The listing builds one solid part. Answer for the finished solid, in the listing's coordinates (mm). Face numbers are marked on the shaded views. A direction names the side the tool comes from. Round coordinates to 2 decimals unless told otherwise and drop trailing zeros. Write each loop counter-clockwise with the first axis right and the second up, starting at its lowest first coordinate (ties: lowest second). Pieces come first, ordered by that corner, then holes. Notation, with made-up numbers: (34, 75.25) - (55, 75.25) arc R6 ccw to (55, 85.25) - close; hole circle Ø8 at (-3, 50). An arc over 180 degrees is marked (long way). Return JSON: item names as keys, results as strings. Group by question number.
(1) Section C-C, the plane x = 14.5 is taken. Write down the section's boundary in (y, z).
(2) Determine the mould class of the marked faces 3, 4, 5 and 6 for opening direction Z: +Z half, -Z half, draft (parallel to the pull), parting line (faces both ways), or undercut.
(3) Find the intervals of material crossed by line 1 along X through (y, z) = (-4.5, -2.5); line 2 along Y through (x, z) = (13, 1.25), in increasing order. Write a range as [from, to].
(4) Section A-A, the plane y = -3 is taken. Give the number of separate pieces and of enclosed holes in the cut face, then the cut area to 3 significant figures.
(5) Section D-D, the plane z = 6 is taken. Write down the section's boundary in (x, y), then the cut area to 3 significant figures.
(6) Section B-B, the plane z = 0 is taken. Write down the section's boundary in (x, y), then the cut area to 3 significant figures.
(7) Which of the six approach directions +Z, -Z, +X, -X, +Y, -Y give full straight-line access (tool end or side, diameter ignored) to the marked faces 1 and 2?
```python
from build123d import *

# Parameters (mm, degrees)
SKETCH2_W           = 42
SKETCH2_H           = 17.8
BOSS_EXTRUDE1_DEPTH = 2
SKETCH3_W           = 2
SKETCH3_H           = 17.8
BOSS_EXTRUDE2_DEPTH = 10
BOSS_EXTRUDE3_DEPTH = 2
SKETCH5_R           = 2.5
CUT_EXTRUDE1_DEPTH  = 2
SKETCH6_R           = 1.25
CUT_EXTRUDE2_DEPTH  = 2


with BuildPart() as part:
    # Sketch2 → Boss-Extrude1 (new body)
    with BuildSketch(Plane(origin=(0, 0, 0), x_dir=(1, 0, 0), z_dir=(0, 1, 0))):
        Rectangle(SKETCH2_W, SKETCH2_H)
    extrude(amount=BOSS_EXTRUDE1_DEPTH)

    # Sketch3 → Boss-Extrude2 (add)
    with BuildSketch(Plane.XZ):
        with Locations((-20, 0)):
            Rectangle(SKETCH3_W, SKETCH3_H)
        with Locations((20, 0)):
            Rectangle(SKETCH3_W, SKETCH3_H)
    extrude(amount=BOSS_EXTRUDE2_DEPTH)

    # Sketch4 → Boss-Extrude3 (add)
    with BuildSketch(Plane.XY.offset(8.9)):
        Polygon((-19, 0), (-14, 0), (-19, -5), align=None)
        Polygon((19, -5), (14, 0), (19, 0), align=None)
    boss_extrude3 = extrude(amount=-BOSS_EXTRUDE3_DEPTH)

    # Mirror1: Boss-Extrude3 across plane
    add(boss_extrude3.mirror(Plane.XY))

    # Sketch5 → Cut-Extrude1 (cut)
    with BuildSketch(Plane.XZ):
        with Locations((-8.319906625, 0)):
            Circle(SKETCH5_R)
        with Locations((6.680093375, 0)):
            Circle(SKETCH5_R)
    extrude(amount=-CUT_EXTRUDE1_DEPTH, mode=Mode.SUBTRACT)

    # Sketch6 → Cut-Extrude2 (cut)
    with BuildSketch(Plane(origin=(-19, 0, 0), x_dir=(0, 0, -1), z_dir=(1, 0, 0))):
        with Locations((-4, -3)):
            Circle(SKETCH6_R)
        with Locations((4, -3)):
            Circle(SKETCH6_R)
    cut_extrude2 = extrude(amount=-CUT_EXTRUDE2_DEPTH, mode=Mode.SUBTRACT)

    # Mirror2: Cut-Extrude2 across plane
    add(cut_extrude2.mirror(Plane(origin=(0, 0, 0), x_dir=(0, 0, 1), z_dir=(1, 0, 0))), mode=Mode.SUBTRACT)


solid = part.part
```
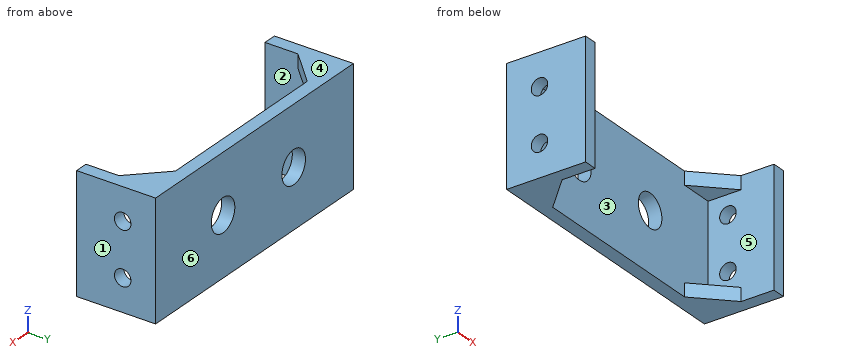
Working result:
{
 "1": {"outline": "(-0.5, -8.9) - (2, -8.9) - (2, 8.9) - (-0.5, 8.9) - (-0.5, 6.9) - (0, 6.9) - (0, -6.9) - (-0.5, -6.9) - close"},
 "2": {"face 3": "undercut", "face 4": "+Z half", "face 5": "undercut", "face 6": "draft"},
 "3": {"line 1": "x = [-21, -19], [19, 21]", "line 2": "y = [0, 2]"},
 "4": {"separate pieces": "6", "enclosed holes": "0", "area": "67.2 mm^2"},
 "5": {"outline": "(-21, -10) - (-19, -10) - (-19, 0) - (19, 0) - (19, -10) - (21, -10) - (21, 2) - (-21, 2) - close", "area": "124 mm^2"},
 "6": {"outline": "(-21, -10) - (-19, -10) - (-19, 0) - (-10.82, 0) - (-10.82, 2) - (-21, 2) - close; (-5.82, 0) - (4.18, 0) - (4.18, 2) - (-5.82, 2) - close; (9.18, 0) - (19, 0) - (19, -10) - (21, -10) - (21, 2) - (9.18, 2) - close", "area": "104 mm^2"},
 "7": {"face 1": "+Z, -Z, +X, +Y, -Y", "face 2": "-Y"}
}
